Source: three-view drawing plus pictorial views. Frame: mm from the lowest corner of the part. Round coordinates to 2 decimals unless told otherwise and drop trailing zeros. Order: outer loops, then holes, each group sorted by start corner. A loop starts at its lowest first (then second) coordinate and runs counter-clockwise, first axis right, second up. Notation, with made-up numbers: (-27.75, 65.25) -> (19.25, 65.25) arc R18 cw to (19.25, 96.25) -> close; hole circle Ø9 at (-29.75, -20). An arc over 180 degrees is marked (long way). Answer as CSV lines item,"result". Start each with the question number.
1) Line query: L1, parallel to Y at x = 3.25, z = 11.5; L2, parallel to Z at x = 8, y = 42; L3, parallel to X at y = 27.5, z = 7.5. Output: solid intervals per line, ascending.
2) Section query A-A, the plane y = 43.5. Output: boundary loops of the cut face in (x, z), and give its area (3 significant figures).
3) Section query B-B, the plane y = 24.5. Output: boundary loops of the cut face in (x, z).
4) First-contact query: P1, Ø6, axis at x = 3.5, y = 32.5, coming from the -Z side; P2, Ø2, axis at x = 3, y = 29, coming from the +Z side; P3, Ø3, axis at x = 11, y = 13.5, coming from the -Z side. Flat tips, straight axial feed; report the tip coordinate or a pass-through.
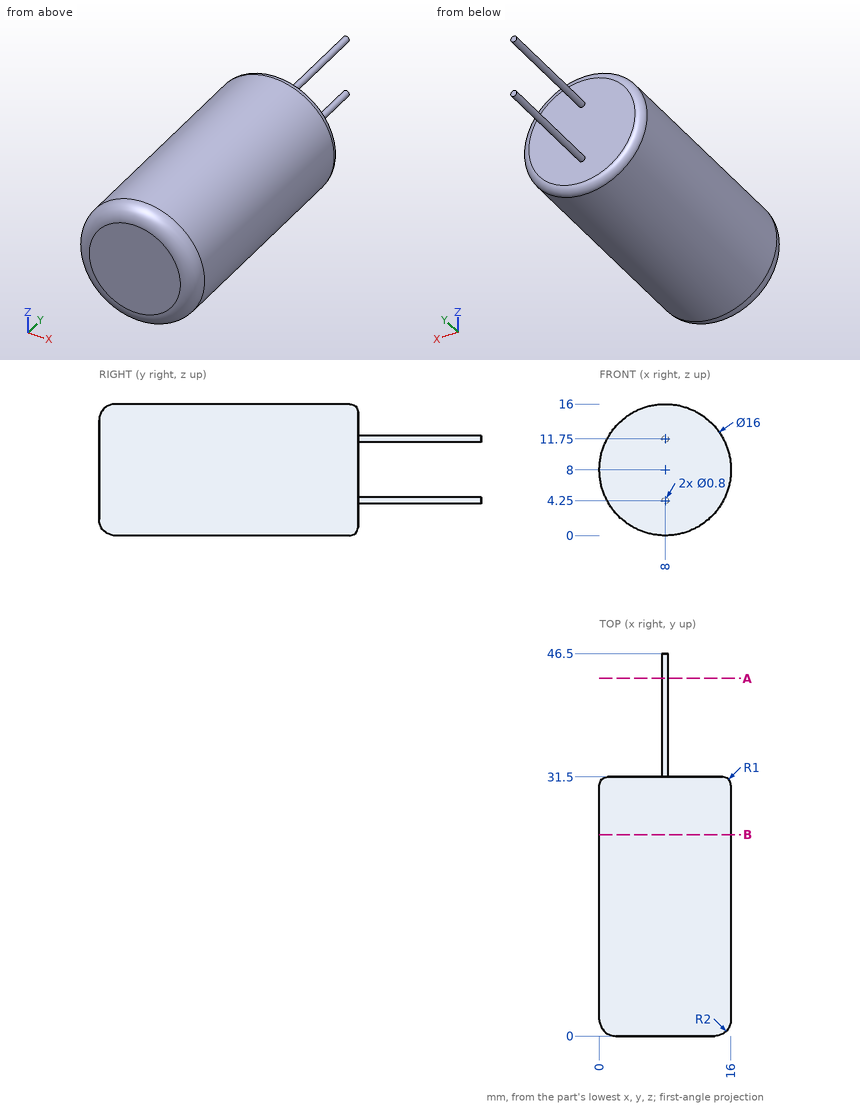
Findings:
1,L1,"y = 0 to 31.5"
1,L2,"z = 3.85 to 4.65, 11.35 to 12.15"
1,L3,"x = 0.02 to 15.98"
2,outline,"circle Ø0.8 at (8, 4.25); circle Ø0.8 at (8, 11.75)"
2,area,"1.01 mm^2"
3,outline,"circle Ø16 at (8, 8)"
4,P1,"stops at z = 0.3"
4,P2,"stops at z = 14.93"
4,P3,"stops at z = 0.14"
